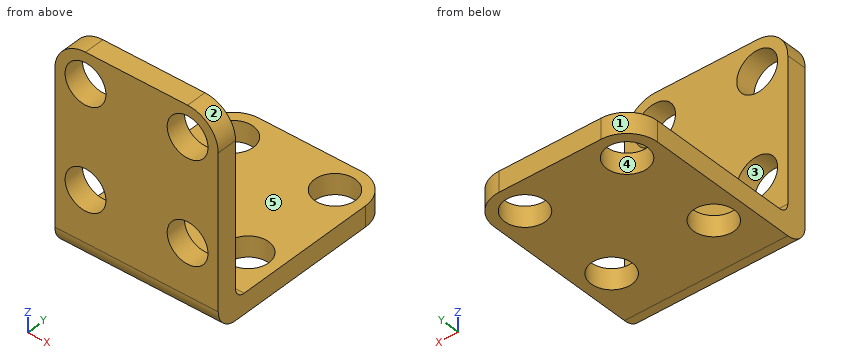
from build123d import *

# Parameters (mm, degrees)
SKETCH_6_W      = 40
SKETCH_6_H      = 50
EXTRUDE_7_DEPTH = 5
SKETCH_12_W     = 40
SKETCH_12_H     = 5
EXTRUDE_8_DEPTH = 45
FILLET_9_R      = 2.5
FILLET_10_R     = 5
MM_2_D          = 10
FILLET_11_R     = 7.5
MM_3_D          = 10


with BuildPart() as part:
    # 草图6 → 凸台-拉伸7 (new body)
    with BuildSketch(Plane.XY):
        Rectangle(SKETCH_6_W, SKETCH_6_H)
    extrude(amount=EXTRUDE_7_DEPTH)

    # 草图12 → 凸台-拉伸8 (add)
    with BuildSketch(Plane.XY.offset(5)):
        with Locations((0, -22.5)):
            Rectangle(SKETCH_12_W, SKETCH_12_H)
    extrude(amount=EXTRUDE_8_DEPTH)

    # 圆角9
    fillet_9_edges = [part.edges().sort_by_distance(p)[0] for p in [
        (0, -20, 5),
    ]]
    fillet(fillet_9_edges, radius=FILLET_9_R)

    # 圆角10
    fillet_10_edges = [part.edges().sort_by_distance(p)[0] for p in [
        (0, -25, 0),
    ]]
    fillet(fillet_10_edges, radius=FILLET_10_R)

    # 大小mm 暗销孔2 (through all)
    with Locations(Plane.XY.offset(5)):
        with Locations((-12.5, 17.5), (-12.5, -7.5), (12.5, -7.5), (12.5, 17.5)):
            Hole(MM_2_D / 2)

    # 圆角11
    fillet_11_edges = [part.edges().sort_by_distance(p)[0] for p in [
        (-20, -22.5, 50),
        (20, -22.5, 50),
        (-20, 25, 2.5),
        (20, 25, 2.5),
    ]]
    fillet(fillet_11_edges, radius=FILLET_11_R)

    # 大小mm 暗销孔3 (through all)
    with Locations(Plane(origin=(0, -20, 0), x_dir=(1, 0, 0), z_dir=(0, 1, 0))):
        with Locations((-12.5, -17.5), (12.5, -17.5), (12.5, -42.5), (-12.5, -42.5)):
            Hole(MM_3_D / 2)


solid = part.part
Here's how the part is built. I have some questions about the finished solid (model axes, mm). Face numbers are marked on the shaded views. A direction names the side the tool comes from. Coordinates: 2 decimals unless noted, no trailing zeros. Write each loop counter-clockwise with the first axis right and the second up, starting at its lowest first coordinate (ties: lowest second). Pieces come first, ordered by that corner, then holes.
Item 1: On a 3-axis mill with a long thin cutter (end or side, diameter ignored), from which of +Z, -Z, +X, -X, +Y, -Y can I reach the whole of each face in a straight line? I mean the marked faces 4 and 5. Say none if no direction works.
Item 2: I want a section at B-B on z = 45.5. Write out the boundary of the cut face in (x, y), and give its area (3 significant figures).
Item 3: I want a section at D-D on x = 0. Write out the boundary of the cut face in (y, z).
Item 4: Will these pins go through, and if not, where does the flat tip stop? pin 1 (12 mm diameter, centred on x = -4, y = 10, fed in from +Z); pin 2 (13 mm diameter, centred on x = -12.5, z = 42.5, fed in from +Y); pin 3 (9 mm diameter, centred on x = 12.5, y = -7.5, fed in from +Z).
Item 5: If we mould it in two halves opening along Z, with no side actions, what happens to the marked faces 1, 2 and 3? For each: +Z half, -Z half, draft (parallel to the pull), parting line (faces both ways), or undercut.
Item 6: I want a section at A-A on y = -3.5. Write out the boundary of the cut face in (x, z), and give its area (3 significant figures).
Item 7: If I drill on line 1 (X direction, y = -21.35, z = 42.5); line 2 (Z direction, x = 12, y = -22); line 3 (Z direction, x = 8, y = 20.5), over which ranges is the centre line in solid material (lowest first)?
Item 8: I want a section at C-C on x = 15. Write out the boundary of the cut face in (y, z).
Findings below:
1. face 4: +Z, -Z
1. face 5: +Z, +X, -X, +Y
2. outline: (-19.37, -25) - (-16.5, -25) - (-16.5, -20) - (-19.37, -20) - close; (-8.5, -25) - (8.5, -25) - (8.5, -20) - (-8.5, -20) - close; (16.5, -25) - (19.37, -25) - (19.37, -20) - (16.5, -20) - close
2. area: 114 mm2
3. outline: (-25, 5) arc R5 ccw to (-20, 0) - (25, 0) - (25, 5) - (-17.5, 5) arc R2.5 cw to (-20, 7.5) - (-20, 50) - (-25, 50) - close
4. pin 1: stops at z = 5
4. pin 2: stops at y = -20
4. pin 3: passes through
5. face 1: draft
5. face 2: +Z half
5. face 3: undercut
6. outline: (-20, 0) - (-15.5, 0) - (-15.5, 5) - (-20, 5) - close; (-9.5, 0) - (9.5, 0) - (9.5, 5) - (-9.5, 5) - close; (15.5, 0) - (20, 0) - (20, 5) - (15.5, 5) - close
6. area: 140 mm2
7. line 1: x = -20 to -17.5, -7.5 to 7.5, 17.5 to 20
7. line 2: z = 0.42 to 12.53, 22.47 to 37.53, 47.47 to 50
7. line 3: z = 0 to 5
8. outline: (-25, 5) arc R5 ccw to (-20, 0) - (-11.83, 0) - (-11.83, 5) - (-17.5, 5) arc R2.5 cw to (-20, 7.5) - (-20, 13.17) - (-25, 13.17) - close; (-25, 21.83) - (-20, 21.83) - (-20, 38.17) - (-25, 38.17) - close; (-25, 46.83) - (-20, 46.83) - (-20, 49.57) - (-25, 49.57) - close; (-3.17, 0) - (13.17, 0) - (13.17, 5) - (-3.17, 5) - close; (21.83, 0) - (24.57, 0) - (24.57, 5) - (21.83, 5) - close
